The drawing under review shows one solid part. Ordinate dimensions are in mm from its lowest x, y, z. A direction names the side the tool comes from. Round coordinates to 2 decimals unless told otherwise and drop trailing zeros. Write each loop counter-clockwise with the first axis right and the second up, starting at its lowest first coordinate (ties: lowest second). Pieces come first, ordered by that corner, then holes.
Item 1: Add section C-C (z = 12.5). Give the boundary of the cut face in (x, y).
Item 2: Add section B-B (x = 25). Give the boundary of the cut face in (y, z).
Item 3: Add section A-A (y = 10). Give the boundary of the cut face in (x, z), plus the area to 3 significant figures.
Item 4: Machinability: for the marked faces 1 and 2, which of the approach directions +Z, -Z, +X, -X, +Y, -Y give a long, thin tool a straight path to every point of the face, cutting with its end or side? Answer none if there is none.
Item 5: Add section D-D (x = 45). Give the boundary of the cut face in (y, z).
Item 6: To check wall thickness, follow L1, parallel to X at y = 10, z = 11.25; L2, parallel to X at y = 10, z = 25.15; L3, parallel to Y at x = 25, z = 25.15. State the ranges of each line that lie inside material, in increasing order.
Item 7: Clearance check with flat-ended pins moving along their axes: pin 1 Ø7 at (x, y) = (6, 10.5) entering from +Z; pin 2 Ø4 at (x, y) = (23, 11.5) entering from -Z; pin 3 Ø4 at (x, y) = (45, 10) entering from +Z; pin 4 Ø4.5 at (x, y) = (25, 8.5) entering from -Z. State where each tip first meets the part, or that it passes through.
Item 8: Draft analysis for pull direction X (two halves, no side actions). For the marked faces 3, 4 and 5, state which applies: +X half, -X half, draft (parallel to the pull), parting line (faces both ways), or undercut.
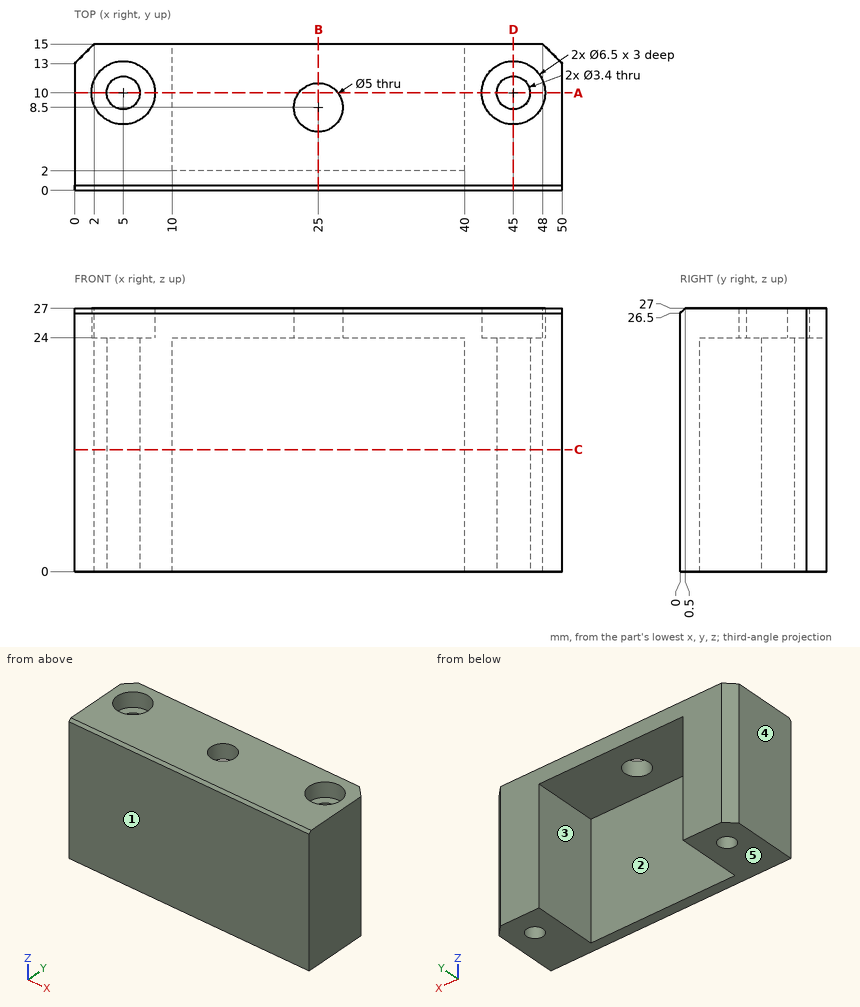
Numbers:
1. outline: (0, 0) - (50, 0) - (50, 13) - (48, 15) - (40, 15) - (40, 2) - (10, 2) - (10, 15) - (2, 15) - (0, 13) - close; hole circle Ø3.4 at (5, 10); hole circle Ø3.4 at (45, 10)
2. outline: (0, 0) - (2, 0) - (2, 24) - (6, 24) - (6, 27) - (0.5, 27) - (0, 26.5) - close; (11, 24) - (15, 24) - (15, 27) - (11, 27) - close
3. outline: (0, 0) - (3.3, 0) - (3.3, 24) - (1.75, 24) - (1.75, 27) - (0, 27) - close; (6.7, 0) - (10, 0) - (10, 24) - (23, 24) - (23, 27) - (8.25, 27) - (8.25, 24) - (6.7, 24) - close; (27, 24) - (40, 24) - (40, 0) - (43.3, 0) - (43.3, 24) - (41.75, 24) - (41.75, 27) - (27, 27) - close; (46.7, 0) - (50, 0) - (50, 27) - (48.25, 27) - (48.25, 24) - (46.7, 24) - close
3. area: 416 mm2
4. face 1: +Z, -Z, +X, -X, -Y
4. face 2: -Z, +Y
5. outline: (0, 0) - (8.3, 0) - (8.3, 24) - (6.75, 24) - (6.75, 27) - (0.5, 27) - (0, 26.5) - close; (11.7, 0) - (15, 0) - (15, 27) - (13.25, 27) - (13.25, 24) - (11.7, 24) - close
6. L1: x = 0 to 3.3, 6.7 to 10, 40 to 43.3, 46.7 to 50
6. L2: x = 0 to 1.75, 8.25 to 23, 27 to 41.75, 48.25 to 50
6. L3: y = 0 to 6, 11 to 15
7. pin 1: stops at z = 27
7. pin 2: stops at z = 24
7. pin 3: stops at z = 24
7. pin 4: passes through
8. face 3: undercut
8. face 4: -X half
8. face 5: draft
